Model file for the job. Use its own axes, mm. Coordinates: 2 decimals unless noted, no trailing zeros. Loops run counter-clockwise (first coordinate to the right, second up) from the corner with the lowest first, then second, coordinate; pieces in that order, holes last. Notation, with made-up numbers: (89.5, 74.5) -> (107.5, 74.5) arc R20 ccw to (107.5, 78.5) -> close; hole circle Ø11 at (-22, -35.5). An arc over 180 degrees is marked (long way). Use one line per item in the form item = value.
Autodesk Inventor part; units mm, degrees
ref_plane "Work Plane1" through (-379.4125, 0, 0) normal (1, 0, 0) x (0, 1, 0)
ref_plane "XZ Plane" through (0, 0, 0) normal (0, 1, 0) x (-1, 0, 0)
ref_plane "XY Plane" through (0, 0, 0) normal (0, 0, 1) x (1, 0, 0)
sketch "Sketch1" plane through (0, 0, 0) normal (0, 1, 0) x (-1, 0, 0)
  line L0 (50.8, 0) -> (733.425, 0)
  line L1 (784.225, -50.8) -> (784.225, -733.425)
  line L2 (733.425, -784.225) -> (50.8, -784.225)
  line L3 (0, -733.425) -> (0, -50.8)
  arc A0 (784.225, -50.8) -> (733.425, 0) centre (733.425, -50.8) ccw
  arc A1 (733.425, -784.225) -> (784.225, -733.425) centre (733.425, -733.425) ccw
  arc A2 (0, -733.425) -> (50.8, -784.225) centre (50.8, -733.425) ccw
  arc A3 (50.8, 0) -> (0, -50.8) centre (50.8, -50.8) ccw
  point P0 (0, 0)
  point P1 (784.225, -784.225)
  point P2 (784.225, 0)
  point P3 (0, -784.225)
  dimension "d0" = 784.225
  dimension "d1" = 784.225
  dimension "d2" = 50.8
ref_plane "Work Plane1" through (-379.4125, 0, 0) normal (1, 0, 0) x (0, 1, 0)
sketch "Sketch2" plane through (-379.4125, 0, 0) normal (1, 0, 0) x (0, 1, 0)
  circle A0 centre (0, 0) radius 25.4
  dimension "d4" = 50.8
sweep "Sweep1" add profiles "Sketch2" path "Sketch1"
properties part number "Pool Noodles"
Q1. Band-saw the part on B-B, the plane z = -368.5. Write the cut outline in (x, y) (3 decimals), and give its area (3 significant figures).
Result:
outline = circle Ø50.8 at (-784.225, 0); circle Ø50.8 at (0, 0)
area = 4,050 mm2
Q2. Pin check, flat tips, straight feed: pin 1 Ø1 at (y, z) = (19, -351.5) entering from +X; pin 2 Ø3 at (y, z) = (-5, -274) entering from -X; pin 3 Ø6 at (y, z) = (-5, -144.5) entering from +X. Stop position of each tip, or through.
Result:
pin_1 = 17.4
pin_2 = -809.38
pin_3 = 25.32
Q3. Wall check: line 1 along Z through (x, y) = (-506, 0) (3 decimals); line 2 along Z through (x, y) = (-454, 4); line 3 along X through (y, z) = (11, -112). Give the ranges that are in metal, low to high.
Result:
line_1 = -809.625 to -758.825, -25.4 to 25.4
line_2 = -809.31 to -759.14, -25.08 to 25.08
line_3 = -807.12 to -761.33, -22.89 to 22.89
Q4. Band-saw the part on C-C, the plane x = -157. Write the cut outline in (y, z) (3 decimals).
Result:
outline = circle Ø50.8 at (0, -784.225); circle Ø50.8 at (0, 0)
Q5. Band-saw the part on A-A, the plane y = 0. Write the cut outline in (x, z) (3 decimals), and give its area (3 significant figures).
Result:
outline = (-809.625, -733.425) arc R76.2 ccw to (-733.425, -809.625) -> (-50.8, -809.625) arc R76.2 ccw to (25.4, -733.425) -> (25.4, -50.8) arc R76.2 ccw to (-50.8, 25.4) -> (-733.425, 25.4) arc R76.2 ccw to (-809.625, -50.8) -> close; hole (-758.825, -733.425) arc R25.4 ccw to (-733.425, -758.825) -> (-50.8, -758.825) arc R25.4 ccw to (-25.4, -733.425) -> (-25.4, -50.8) arc R25.4 ccw to (-50.8, -25.4) -> (-733.425, -25.4) arc R25.4 ccw to (-758.825, -50.8) -> close
area = 155,000 mm2
